Input: part model. Units: mm. Frame: model coordinates. Coordinates: 2 decimals unless noted, no trailing zeros. Order: outer loops, then holes, each group sorted by start corner. A loop starts at its lowest first (then second) coordinate and runs counter-clockwise, first axis right, second up. Notation, with made-up numbers: (46, 89.25) -> (53, 89.25) arc R10 ccw to (53, 93.25) -> close; hole circle Ø2 at (2.5, 13). An arc over 180 degrees is marked (long way). Write each question's results on one line, items separated by ' | '.
```python
from build123d import *

# Parameters (mm, degrees)
F1_DEPTH = 4
F2_R     = 2


with BuildPart() as f1:
    # F0 (on Top) → F1 (new body)
    with BuildSketch(Plane.XY):
        Polygon((-38.920617, 0), (0, 0), (-19.38504, 28), align=None)
    extrude(amount=F1_DEPTH)

    # F2
    f2_edges = [f1.edges().sort_by_distance(p)[0] for p in [
        (-19.38504, 28, 2),
        (-38.920617, 0, 2),
        (0, 0, 2),
    ]]
    fillet(f2_edges, radius=F2_R)


solid = f1.part
```
(1) Cut plane A-A, the plane z = 2.35. Return loops of the section in (x, y), plus the area to 3 significant figures.
Return value:
outline: (-36.73, 3.14) arc R2 ccw to (-35.09, 0) -> (-3.82, 0) arc R2 ccw to (-2.17, 3.14) -> (-17.75, 25.63) arc R2 ccw to (-21.03, 25.64) -> close | area: 536 mm2
(2) Cut plane B-B, the plane x = -9. Return loops of the section in (y, z).
Return value:
outline: (0, 0) -> (13, 0) -> (13, 4) -> (0, 4) -> close
(3) Line query: line 1 along X through (y, z) = (8.5, 3.1); line 2 along X through (y, z) = (15.5, 1.65); line 3 along Y through (x, z) = (-33, 2.4). Output: solid intervals per line, ascending. Write a range as from..to.
Return value:
line 1: -32.99..-5.88 | line 2: -28.11..-10.73 | line 3: 0..8.49
(4) Pin query (flat end, axial travel): P1, Ø2, axis at y = 14, z = 1.5, coming from the -X side. Return the tip coordinate at first contact, or that it passes through.
Return value:
P1: x = -29.85
(5) Cut plane C-C, the plane y = 10.5. Return loops of the section in (x, z).
Return value:
outline: (-31.59, 0) -> (-7.27, 0) -> (-7.27, 4) -> (-31.59, 4) -> close
